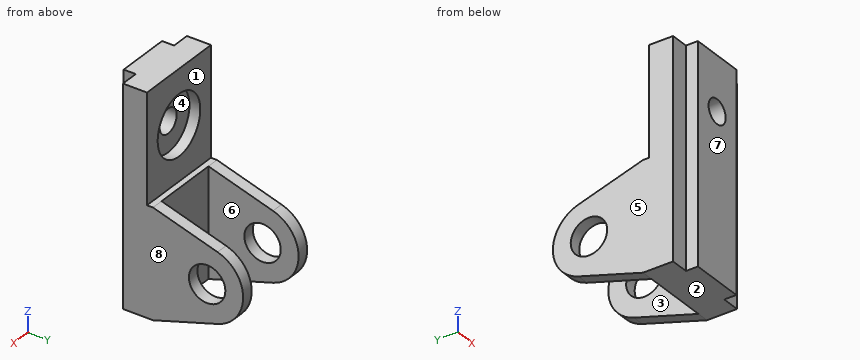
from build123d import *

# Parameters (mm, degrees)
SKETCH1_W           = 75
SKETCH1_H           = 180
BOSS_EXTRUDE1_DEPTH = 30
SKETCH2_W           = 15
SKETCH2_H           = 10
CUT_EXTRUDE1_DEPTH  = 187.296135226
SKETCH3_R           = 15.149621256
BOSS_EXTRUDE2_DEPTH = 75
CUT_EXTRUDE2_START  = 5
SKETCH4_W           = 55
SKETCH4_H           = 90
CUT_EXTRUDE2_DEPTH  = 122.119982556
HOLE1_D             = 20
HOLE1_CBORE_D       = 50
HOLE1_CBORE_DEPTH   = 9


with BuildPart() as part:
    # Sketch1 → Boss-Extrude1 (new body)
    with BuildSketch(Plane(origin=(0, 0, 0), x_dir=(1, 0, 0), z_dir=(0, 1, 0))):
        Rectangle(SKETCH1_W, SKETCH1_H)
    extrude(amount=BOSS_EXTRUDE1_DEPTH)

    # Sketch2 → Cut-Extrude1 (cut, through all)
    with BuildSketch(Plane.XY.offset(90)):
        with Locations((-30, 5)):
            Rectangle(SKETCH2_W, SKETCH2_H)
    cut_extrude1 = extrude(amount=-CUT_EXTRUDE1_DEPTH, mode=Mode.SUBTRACT)

    # Mirror1: Cut-Extrude1 across plane
    add(cut_extrude1.mirror(Plane(origin=(0, 0, 0), x_dir=(0, 0, 1), z_dir=(1, 0, 0))), mode=Mode.SUBTRACT)

    # Sketch3 → Boss-Extrude2 (add)
    with BuildSketch(Plane.ZY.offset(37.5)):
        with BuildLine():
            Line((-90, 30), (-90, 35))
            Line((-90, 35), (-73.708286934, 88.708286934))
            ThreePointArc((-73.708286934, 88.708286934), (-45, 110), (-16.291713066, 88.708286934))
            Line((-16.291713066, 88.708286934), (0, 35))
            Line((0, 35), (0, 30))
            Line((0, 30), (-90, 30))
        make_face()
        with Locations((-45, 80)):
            Circle(SKETCH3_R, mode=Mode.SUBTRACT)
    extrude(amount=-BOSS_EXTRUDE2_DEPTH)

    # Sketch4 → Cut-Extrude2 (cut, through all)
    with BuildSketch(Plane(origin=(0, 30, 0), x_dir=(1, 0, 0), z_dir=(0, 1, 0)).offset(CUT_EXTRUDE2_START)):
        with Locations((0, 45)):
            Rectangle(SKETCH4_W, SKETCH4_H)
    extrude(amount=CUT_EXTRUDE2_DEPTH, mode=Mode.SUBTRACT)

    # Hole1 (through all)
    with Locations(Plane(origin=(0, 30, 0), x_dir=(1, 0, 0), z_dir=(0, 1, 0))):
        with Locations((0, -45)):
            CounterBoreHole(HOLE1_D / 2, HOLE1_CBORE_D / 2, HOLE1_CBORE_DEPTH)


solid = part.part
Source: CAD feature listing. Evaluate the final solid. Frame: model axes, mm. Face numbers are marked on the shaded views. A direction names the side the tool comes from. Coordinates: 2 decimals unless noted, no trailing zeros. Loops run counter-clockwise (first coordinate to the right, second up) from the corner with the lowest first, then second, coordinate; pieces in that order, holes last. Notation, with made-up numbers: (-35.5, 58.5) - (-19.5, 58.5) arc R24 cw to (-19.5, 86.5) - close; hole circle Ø7 at (59.25, 76). An arc over 180 degrees is marked (long way). Return JSON: item names as keys, results as strings.
Q1. Section D-D, the plane z = 2.5. Return loops of the section in (x, y).
Results:
{"outline": "(-37.5, 10) - (-22.5, 10) - (-22.5, 0) - (22.5, 0) - (22.5, 10) - (37.5, 10) - (37.5, 30) - (-37.5, 30) - close"}
Q2. Contact query for flat-ended pins moving along their axis: P1, Ø3, axis at x = -11, z = 22, coming from the +Y side; P2, Ø4.5, axis at x = -33, z = 18.5, coming from the -Y side; P3, Ø5, axis at y = 3.5, z = -28.5, coming from the +X side; P4, Ø24, axis at y = 80, z = -45, coming from the +X side. Output: stop coordinate, or through.
Results:
{"P1": "y = 30", "P2": "y = 10", "P3": "x = 22.5", "P4": "through"}
Q3. Mould query, pull axis X, two halves, no side actions, for the marked faces 5, 6, 7 and 8. Classes: released by +X, released by -X, zero draft, split by the parting line, or undercut.
Results:
{"face 5": "released by -X", "face 6": "undercut", "face 7": "zero draft", "face 8": "released by +X"}
Q4. Access query for the marked faces 1, 2, 3 and 4. Directions: +Z, -Z, +X, -X, +Y, -Y. A direction counts if a zero-diameter tool reaches every point of the face in a straight line with its end or side. Return the directions, or none.
Results:
{"face 1": "+Z, +X, -X, +Y", "face 2": "-Z, +X, -X, +Y, -Y", "face 3": "+Z, -Z, +Y", "face 4": "+Y"}
Q5. Section A-A, the plane z = 45. Return loops of the section in (x, y).
Results:
{"outline": "(-37.5, 10) - (-22.5, 10) - (-22.5, 0) - (-10, 0) - (-10, 21) - (-25, 21) - (-25, 30) - (-37.5, 30) - close; (10, 0) - (22.5, 0) - (22.5, 10) - (37.5, 10) - (37.5, 30) - (25, 30) - (25, 21) - (10, 21) - close"}
Q6. Section C-C, the plane y = 60. Return loops of the section in (x, z).
Results:
{"outline": "(-37.5, -82.42) - (-27.5, -82.42) - (-27.5, -7.58) - (-37.5, -7.58) - close; (27.5, -82.42) - (37.5, -82.42) - (37.5, -7.58) - (27.5, -7.58) - close"}
Q7. Section B-B, the plane x = 0. Return loops of the section in (y, z), plus the area to 3 significant figures.
Results:
{"outline": "(0, -90) - (35, -90) - (35, 0) - (30, 0) - (30, 20) - (21, 20) - (21, 35) - (0, 35) - close; (0, 55) - (21, 55) - (21, 70) - (30, 70) - (30, 90) - (0, 90) - close", "area": "4,980 mm2"}
Q8. Material intervals for line 1 along Z through (x, y) = (0, 27.5); line 2 along X through (y, z) = (92.5, -54); line 3 along Y through (x, z) = (32, -45), sorted ascending.
Results:
{"line 1": "-90 to 20, 70 to 90", "line 2": "-37.5 to -27.5, 27.5 to 37.5", "line 3": "10 to 64.85, 95.15 to 110"}
